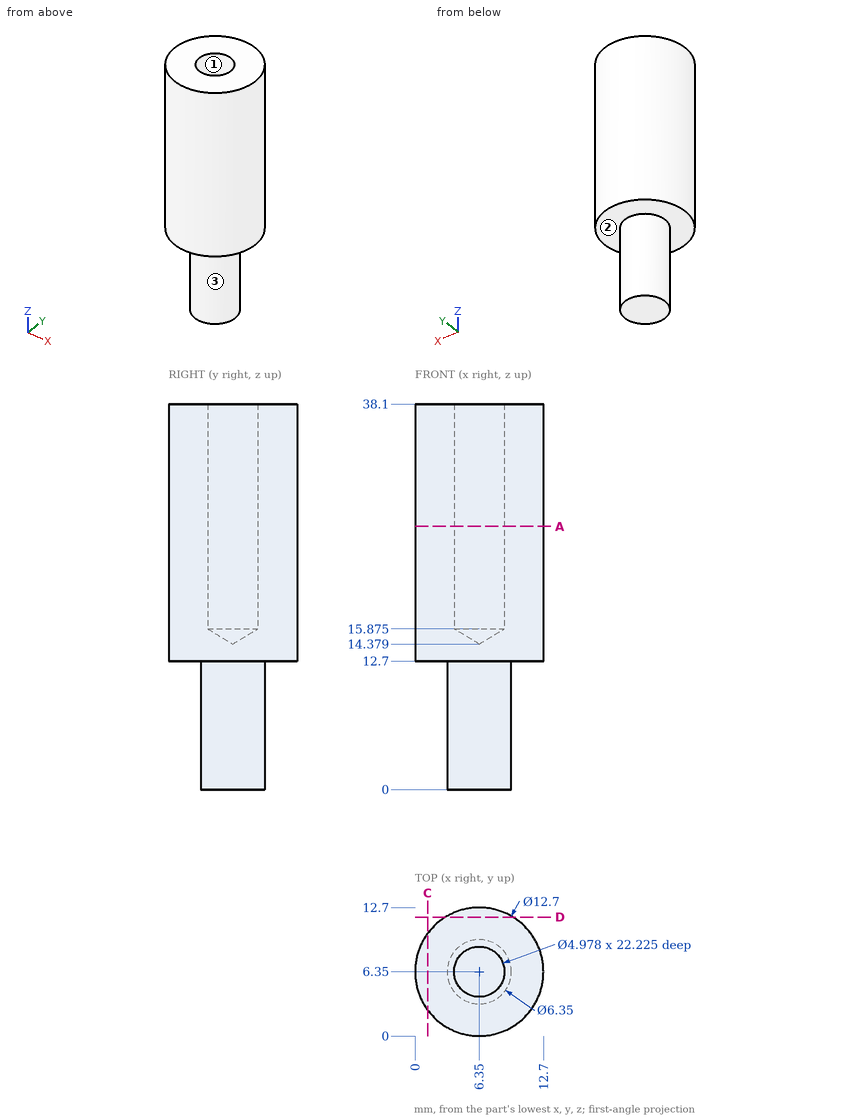
Could you check a few things on this drawing? It's one solid part, dimensions in mm from its lowest x, y, z. Give positions to 0.01 mm unless a question says otherwise; leave off trailing zeros. Order: outer loops, then holes, each group sorted by start corner. A loop starts at its lowest first (then second) coordinate and runs counter-clockwise, first axis right, second up. Notation, with made-up numbers: (47, 49) - (85, 49) arc R22 cw to (85, 70) - close; hole circle Ø6 at (67, 5.5). An arc over 180 degrees is marked (long way). Answer as a JSON object with one key per item and string values. Group by question number.
Item 1: If we section it at A-A on z = 26: Please give me the cut outline in (x, y), and give its area (3 significant figures).
Item 2: Please list where these lines run through material, in increasing order: probe 1 along Y at (x, z) = (6.35, 24); probe 2 along Z at (x, y) = (10.5, 4.25); probe 3 along Y at (x, z) = (6.5, 6.5).
Item 3: If we mould it in two halves opening along Y, with no side actions, what happens to the marked faces 1, 2 and 3? For each: pulls with the +Y half, pulls with the -Y half, needs draft (parallel to the pull), parting line crosses it, or undercut.
Item 4: If we section it at C-C on x = 1.25: Please give me the cut outline in (y, z).
Item 5: If we section it at D-D on y = 11.75: Please give me the cut outline in (x, z).
Item 6: For P1, Ø4, axis at y = 4, z = 23, coming from the -X side; P2, Ø3, axis at y = 9, z = 23.5, coming from the +X side (1 decimal); P3, Ø6, axis at y = 3.5, z = 9, coming from the -X side (3 decimals), each with a flat end and sliding along its axis, tell me the tip position at first contact or that it passes through.
Result set:
{
 "1": {"outline": "circle Ø12.7 at (6.35, 6.35); hole circle Ø4.98 at (6.35, 6.35)", "area": "107 mm²"},
 "2": {"probe 1": "0 to 3.86, 8.84 to 12.7", "probe 2": "12.7 to 38.1", "probe 3": "3.18 to 9.52"},
 "3": {"face 1": "undercut", "face 2": "needs draft", "face 3": "parting line crosses it"},
 "4": {"outline": "(2.57, 12.7) - (10.13, 12.7) - (10.13, 38.1) - (2.57, 38.1) - close"},
 "5": {"outline": "(3.01, 12.7) - (9.69, 12.7) - (9.69, 38.1) - (3.01, 38.1) - close"},
 "6": {"P1": "x = 0.01", "P2": "x = 12.6", "P3": "x = 3.175"}
}
